from build123d import *

# Parameters (mm, degrees)
SKETCH1_W           = 30
SKETCH1_H           = 40
SKETCH1_R           = 2
BOSS_EXTRUDE1_DEPTH = 1.5
CHAMFER1_SIZE       = 8
SKETCH2_W           = 10
SKETCH2_H           = 10
BOSS_EXTRUDE2_DEPTH = 1.5
CHAMFER3_SIZE       = 1
FILLET1_R           = 3


with BuildPart() as part:
    # Sketch1 → Boss-Extrude1 (new body)
    with BuildSketch(Plane.XY):
        with Locations((15, -20)):
            Rectangle(SKETCH1_W, SKETCH1_H)
        with Locations((20, -34)):
            Circle(SKETCH1_R, mode=Mode.SUBTRACT)
        with Locations((10, -34)):
            Circle(SKETCH1_R, mode=Mode.SUBTRACT)
        with Locations((20, -24)):
            Circle(SKETCH1_R, mode=Mode.SUBTRACT)
        with Locations((10, -24)):
            Circle(SKETCH1_R, mode=Mode.SUBTRACT)
    extrude(amount=BOSS_EXTRUDE1_DEPTH)

    # Chamfer1
    chamfer1_edges = [part.edges().sort_by_distance(p)[0] for p in [
        (0, 0, 0.75),
        (30, 0, 0.75),
        (30, -40, 0.75),
        (0, -40, 0.75),
    ]]
    chamfer(chamfer1_edges, length=CHAMFER1_SIZE)

    # Sketch2 → Boss-Extrude2 (add)
    with BuildSketch(Plane.XY.offset(1.5)):
        with Locations((7.5, -0.5)):
            Rectangle(SKETCH2_W, SKETCH2_H)
    extrude(amount=-BOSS_EXTRUDE2_DEPTH)

    # Chamfer3
    chamfer3_edges = [part.edges().sort_by_distance(p)[0] for p in [
        (12.5, 4.5, 0.75),
        (2.5, 4.5, 0.75),
    ]]
    chamfer(chamfer3_edges, length=CHAMFER3_SIZE)

    # Fillet1
    fillet1_edges = [part.edges().sort_by_distance(p)[0] for p in [
        (12.5, 0, 0.75),
    ]]
    fillet(fillet1_edges, radius=FILLET1_R)


solid = part.part
Read the model definition and answer for the solid it produces. Units are mm, in the model's axes. A direction names the side the tool comes from. Round coordinates to 2 decimals unless told otherwise and drop trailing zeros. Order: outer loops, then holes, each group sorted by start corner. A loop starts at its lowest first (then second) coordinate and runs counter-clockwise, first axis right, second up.
1) The part is cut by section D-D on x = 23.5. Write down the section's boundary in (y, z), plus the area to 3 significant figures.
2) The mould has two halves that part along Y. Classify faces 1 (the face through (4, -36, 1)), 2 (the face through (3, 4, 1)), 3 (the face through (18.526, -22.648, 0.74)): released by +Y, released by -Y, zero draft, split by the parting line, or undercut.
3) The part is cut by section B-B on z = 1.2. Write down the section's boundary in (x, y), plus the area to 3 significant figures.
4) A flat-ended cylindrical pin translates along its axis: pin 1 (0.6 mm diameter, centred on y = 3.5, z = 1, fed in from +X). Find the tip coordinate at first contact, or state that the pin passes through.
5) Straight lines are drawn through the part: L1, parallel to Y at x = 20, z = 1.15; L2, parallel to Y at x = 10, z = 1; L3, parallel to Y at x = 17.5, z = 0.75. For each, find the intervals that lie inside material, in ascending order.
6) The part is cut by section A-A on y = -34. Write down the section's boundary in (x, z), plus the area to 3 significant figures.
7) For faces 4 (the face through (19, 0, 1)), 5 (the face through (15, -17, 0)), 6 (the face through (2.5, -1, 1)), determine the directions among +Z, -Z, +X, -X, +Y, -Y from which every point of the face is accessible in a straight line to the end or side of a thin tool.
8) The part is cut by section C-C on x = 10. Write down the section's boundary in (y, z), plus the area to 4 significant figures.
Resolved:
1. outline: (-38.5, 0) - (-1.5, 0) - (-1.5, 1.5) - (-38.5, 1.5) - close
1. area: 55.5 mm2
2. face 1: released by -Y
2. face 2: released by +Y
2. face 3: undercut
3. outline: (0, -32) - (8, -40) - (22, -40) - (30, -32) - (30, -8) - (22, 0) - (15.5, 0) arc R3 cw to (12.5, 3) - (12.5, 3.5) - (11.5, 4.5) - (3.5, 4.5) - (2.5, 3.5) - (2.5, -5.5) - (0, -8) - close; hole circle Ø4 at (10, -34); hole circle Ø4 at (10, -24); hole circle Ø4 at (20, -34); hole circle Ø4 at (20, -24)
3. area: 1,080 mm2
4. pin 1: stops at x = 12.5
5. L1: y = -40 to -36, -32 to -26, -22 to 0
5. L2: y = -40 to -36, -32 to -26, -22 to 4.5
5. L3: y = -40 to 0
6. outline: (2, 0) - (8, 0) - (8, 1.5) - (2, 1.5) - close; (12, 0) - (18, 0) - (18, 1.5) - (12, 1.5) - close; (22, 0) - (28, 0) - (28, 1.5) - (22, 1.5) - close
6. area: 27.0 mm2
7. face 4: +Z, -Z, +X, +Y
7. face 5: -Z, +X, -X, +Y, -Y
7. face 6: +Z, -Z, -X, +Y
8. outline: (-40, 0) - (-36, 0) - (-36, 1.5) - (-40, 1.5) - close; (-32, 0) - (-26, 0) - (-26, 1.5) - (-32, 1.5) - close; (-22, 0) - (4.5, 0) - (4.5, 1.5) - (-22, 1.5) - close
8. area: 54.75 mm2
